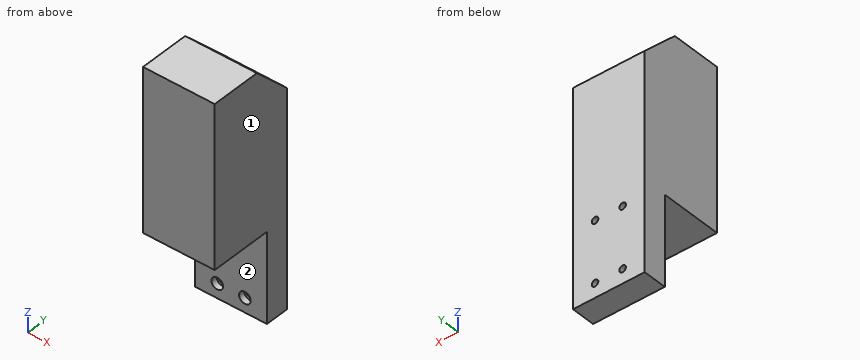
```python
from build123d import *

# Parameters (mm, degrees)
F0_W           = 60
F0_H           = 210
F1_DEPTH       = 72
F2_W           = 52
F2_H           = 75
F3_DEPTH       = 60.001
F4_SIZE        = 30
F7_D           = 5.5
F7_CBORE_D     = 9.75
F7_CBORE_DEPTH = 5


with BuildPart() as f1:
    # F0 (on Front) → F1 (new body)
    with BuildSketch(Plane.XZ):
        Rectangle(F0_W, F0_H)
    extrude(amount=F1_DEPTH)

    # F2 (on face) → F3 (cut, through all)
    with BuildSketch(Plane.YZ.offset(30)):
        with Locations((-46, -67.5)):
            Rectangle(F2_W, F2_H)
    extrude(amount=-F3_DEPTH, mode=Mode.SUBTRACT)

    # F4
    f4_edges = [f1.edges().sort_by_distance(p)[0] for p in [
        (0, 0, 105),
    ]]
    chamfer(f4_edges, length=F4_SIZE)

    # F7 (through all)
    with Locations(Plane.XZ.offset(20)):
        with Locations((-11.5400338545, -42), (11.5400338545, -42), (-11.5400338545, -93), (11.5400338545, -93)):
            CounterBoreHole(F7_D / 2, F7_CBORE_D / 2, F7_CBORE_DEPTH)


solid = f1.part
```
Input: part model. Units: mm. Frame: model coordinates. Face numbers are marked on the shaded views. A direction names the side the tool comes from. Give positions to 0.01 mm unless a question says otherwise; leave off trailing zeros. Order: outer loops, then holes, each group sorted by start corner. A loop starts at its lowest first (then second) coordinate and runs counter-clockwise, first axis right, second up. Notation, with made-up numbers: (84, -1) - (90, -1) arc R34 ccw to (90, 32) - close; hole circle Ø11 at (30.25, -23). An arc over 180 degrees is marked (long way). One line per item, written item: value.
1. Cut plane D-D, the plane z = -55. Output: boundary loops of the cut face in (x, y), and give its area (3 significant figures).
Determined:
outline: (-30, -20) - (30, -20) - (30, 0) - (-30, 0) - close
area: 1,200 mm2
2. Reachability of the marked faces 1 and 2 from +Z, -Z, +X, -X, +Y, -Y: full face, straight path, thin tool, end or side. Return the list, or none.
Determined:
face 1: +Z, -Z, +X, +Y, -Y
face 2: -Z, +X, -X, -Y
3. Line query: probe 1 along Z at (x, y) = (-21.5, -64); probe 2 along Y at (x, z) = (5, -69); probe 3 along Z at (x, y) = (-11, -8). Output: solid intervals per line, ascending.
Determined:
probe 1: -30 to 105
probe 2: -20 to 0
probe 3: -105 to -95.7, -90.3 to -44.7, -39.3 to 83
4. Cut plane C-C, the plane x = 18.5. Output: boundary loops of the cut face in (y, z).
Determined:
outline: (-72, -30) - (-20, -30) - (-20, -105) - (0, -105) - (0, 75) - (-30, 105) - (-72, 105) - close
5. Cut plane A-A, the plane z = -93. Output: boundary loops of the cut face in (x, y).
Determined:
outline: (-30, -20) - (-16.42, -20) - (-16.42, -15) - (-14.29, -15) - (-14.29, 0) - (-30, 0) - close; (-8.79, -15) - (-6.67, -15) - (-6.67, -20) - (6.67, -20) - (6.67, -15) - (8.79, -15) - (8.79, 0) - (-8.79, 0) - close; (14.29, -15) - (16.42, -15) - (16.42, -20) - (30, -20) - (30, 0) - (14.29, 0) - close
6. Pin query (flat end, axial travel): pin 1 Ø4 at (x, y) = (21, -43) entering from -Z; pin 2 Ø9 at (x, z) = (11.54, -93) entering from -Y; pin 3 Ø8 at (x, z) = (14, 80) entering from +Y; pin 4 Ø4.5 at (x, z) = (-11.54, -42) entering from -Y. Return the tip coordinate at first contact, or that it passes through.
Determined:
pin 1: z = -30
pin 2: y = -15
pin 3: y = -1
pin 4: through
7. Cut plane B-B, the plane y = -8.5. Output: boundary loops of the cut face in (x, z).
Determined:
outline: (-30, -105) - (30, -105) - (30, 83.5) - (-30, 83.5) - close; hole circle Ø5.5 at (-11.54, -93); hole circle Ø5.5 at (-11.54, -42); hole circle Ø5.5 at (11.54, -93); hole circle Ø5.5 at (11.54, -42)
